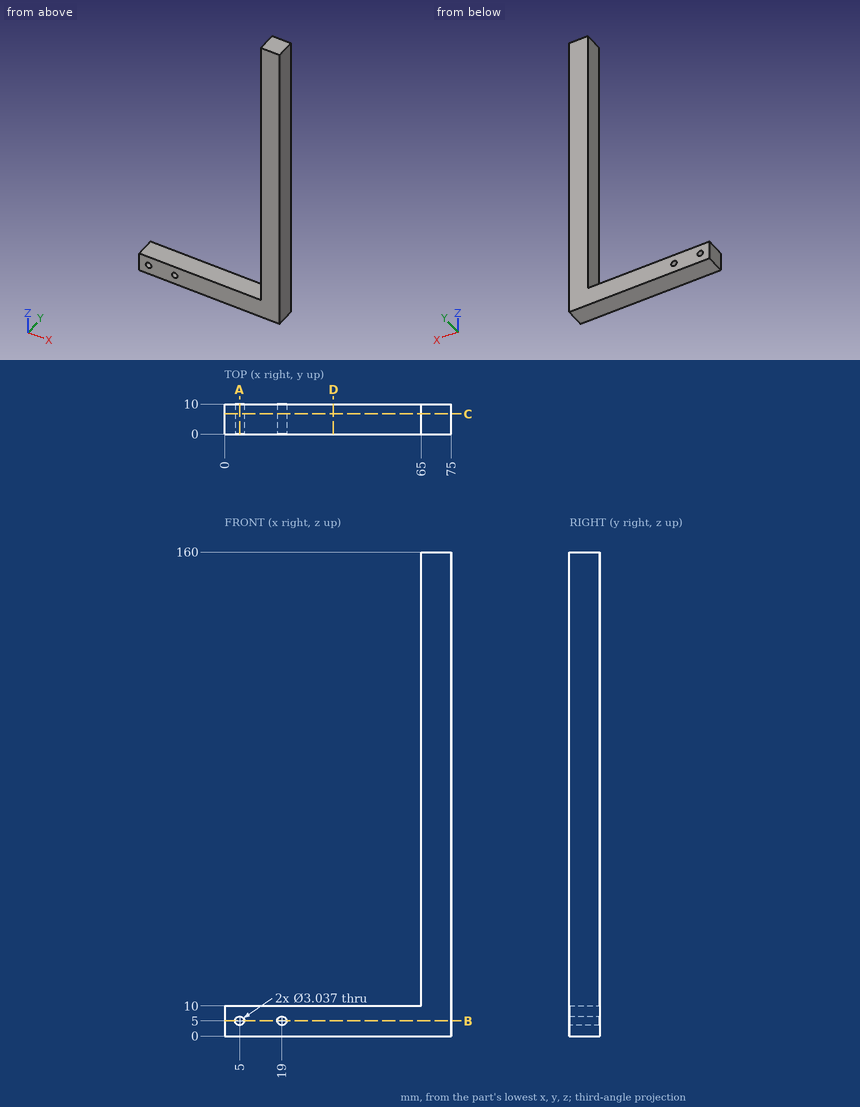
Print and shaded views of the part. All mm, measured from the part's lowest x, y and z. Coordinates: 2 decimals unless noted, no trailing zeros. Order: outer loops, then holes, each group sorted by start corner. A loop starts at its lowest first (then second) coordinate and runs counter-clockwise, first axis right, second up.
(1) Slice it at D-D, the plane x = 36. Write the cut outline in (y, z), and give its area (3 significant figures).
Check sheet entries:
outline: (0, 0) - (10, 0) - (10, 10) - (0, 10) - close
area: 100 mm2
(2) Slice it at A-A, the plane x = 5. Write the cut outline in (y, z).
Check sheet entries:
outline: (0, 0) - (10, 0) - (10, 3.48) - (0, 3.48) - close; (0, 6.52) - (10, 6.52) - (10, 10) - (0, 10) - close
(3) Slice it at C-C, the plane y = 6.75. Write the cut outline in (x, z), and give its area (3 significant figures).
Check sheet entries:
outline: (0, 0) - (75, 0) - (75, 160) - (65, 160) - (65, 10) - (0, 10) - close; hole circle Ø3.04 at (5, 5); hole circle Ø3.04 at (19, 5)
area: 2,240 mm2
(4) Probe L1, parallel to X at y = 4.75, z = 5; L2, parallel to Z at x = 51, y = 8.25; L3, parallel to X at y = 7, z = 46.5. List the from-to ranges inside material, lowest first.
Check sheet entries:
L1: x = 0 to 3.48, 6.52 to 17.48, 20.52 to 75
L2: z = 0 to 10
L3: x = 65 to 75
(5) Slice it at B-B, the plane z = 5. Write the cut outline in (x, y), and give its area (3 significant figures).
Check sheet entries:
outline: (0, 0) - (3.48, 0) - (3.48, 10) - (0, 10) - close; (6.52, 0) - (17.48, 0) - (17.48, 10) - (6.52, 10) - close; (20.52, 0) - (75, 0) - (75, 10) - (20.52, 10) - close
area: 689 mm2
(6) Pin check, flat tips, straight feed: pin 1 Ø2.5 at (x, z) = (5, 5) entering from +Y; pin 2 Ø5 at (x, y) = (62, 6) entering from -Z; pin 3 Ø3 at (x, y) = (17.5, 6.5) entering from +Z; pin 4 Ø3 at (y, z) = (3.5, 93.5) entering from -X. Stop position of each tip, or through.
Check sheet entries:
pin 1: passes through
pin 2: stops at z = 0
pin 3: stops at z = 10
pin 4: stops at x = 65
